Could you check a few things on this model? Use its own coordinates, in mm. A direction names the side the tool comes from. Coordinates: 2 decimals unless noted, no trailing zeros. Order: outer loops, then holes, each group sorted by start corner. A loop starts at its lowest first (then second) coordinate and runs counter-clockwise, first axis right, second up. Notation, with made-up numbers: (73.25, 15) -> (92.25, 15) arc R28 cw to (92.25, 41) -> close; hole circle Ø6 at (26, 85.25). An arc over 180 degrees is marked (long way). Return JSON: item names as keys, results as strings. Group by question number.
from build123d import *

# Parameters (mm, degrees)
F2_R    = 5.08
F3_SIZE = 5.08
F4_SIZE = 5.08


with BuildPart() as f1:
    # F0 (on Front) → F1 (revolve)
    with BuildSketch(Plane.XZ):
        Polygon((12.7, 25.4), (0, 25.4), (0, -6.35), (130.3428560495, -6.35), (279.4, -6.35), (279.4, 25.4), (266.7, 25.4), (266.7, 0), (12.7, 0), align=None)
    revolve(axis=Axis((139.7, 0, -6.35), (-1, 0, 0)))

    # F2
    f2_edges = [f1.edges().sort_by_distance(p)[0] for p in [
        (12.7, 0, -12.7),
        (266.7, 0, -12.7),
    ]]
    fillet(f2_edges, radius=F2_R)

    # F3
    f3_edges = [f1.edges().sort_by_distance(p)[0] for p in [
        (12.7, 0, -38.1),
    ]]
    chamfer(f3_edges, length=F3_SIZE)

    # F4
    f4_edges = [f1.edges().sort_by_distance(p)[0] for p in [
        (266.7, 0, -38.1),
    ]]
    chamfer(f4_edges, length=F4_SIZE)


solid = f1.part
Q1. On a 3-axis mill with a long thin cutter (end or side, diameter ignored), from which of +Z, -Z, +X, -X, +Y, -Y can I reach the whole of each face in a straight line? I mean faces 1 (the flat face through (279.4, 0, -6)), 2 (the cylindrical face through (137.993, 1.907, -0.293)). Say none if no direction works.
Q2. I want a section at A-A on y = 0. Please give me the cut outline in (x, z), and give its area (3 significant figures).
Q3. I want a section at C-C on x = 170. Please give me the cut outline in (y, z), and give its area (3 significant figures).
Q4. I need wall thicknesses on line 1 along X through (y, z) = (14.5, -5); line 2 along X through (y, z) = (27, -18); line 3 along Z through (x, y) = (229.5, -1.5). Which ranges of each line are inside material? Lowest first, please. Write a range as from..to.
Q5. I want a section at B-B on z = -6.35. Please give me the cut outline in (x, y), and give its area (3 significant figures).
Q6. I'm going to push a flat-ended pin straight in: pin 1 Ø3 at (x, y) = (147.5, -1.5) entering from -Z. Where does the tip first touch, or does it pass through?
Response values:
{
 "1": {"face 1": "+Z, -Z, +X, +Y, -Y", "face 2": "none"},
 "2": {"outline": "(0, -38.1) -> (7.62, -38.1) -> (12.7, -33.02) -> (12.7, -17.78) arc R5.08 cw to (17.78, -12.7) -> (261.62, -12.7) arc R5.08 cw to (266.7, -17.78) -> (266.7, -33.02) -> (271.78, -38.1) -> (279.4, -38.1) -> (279.4, 25.4) -> (271.78, 25.4) -> (266.7, 20.32) -> (266.7, 5.08) arc R5.08 cw to (261.62, 0) -> (17.78, 0) arc R5.08 cw to (12.7, 5.08) -> (12.7, 20.32) -> (7.62, 25.4) -> (0, 25.4) -> close", "area": "4,810 mm²"},
 "3": {"outline": "circle Ø12.7 at (0, -6.35)", "area": "127 mm²"},
 "4": {"line 1": "x = 0..12.7, 266.7..279.4", "line 2": "x = 0..9.96, 269.44..279.4", "line 3": "z = -12.52..-0.18"},
 "5": {"outline": "(0, -31.75) -> (7.62, -31.75) -> (12.7, -26.67) -> (12.7, -11.43) arc R5.08 cw to (17.78, -6.35) -> (261.62, -6.35) arc R5.08 cw to (266.7, -11.43) -> (266.7, -26.67) -> (271.78, -31.75) -> (279.4, -31.75) -> (279.4, 31.75) -> (271.78, 31.75) -> (266.7, 26.67) -> (266.7, 11.43) arc R5.08 cw to (261.62, 6.35) -> (17.78, 6.35) arc R5.08 cw to (12.7, 11.43) -> (12.7, 26.67) -> (7.62, 31.75) -> (0, 31.75) -> close", "area": "4,810 mm²"},
 "6": {"pin 1": "stops at z = -12.7"}
}
